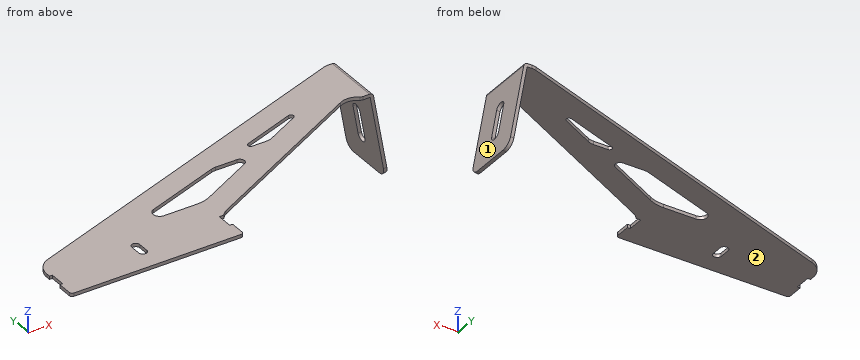
Autodesk Inventor part; units mm, degrees
ref_plane "工作平面1" through (65, 2, 0) normal (-1, 0, 0) x (0, 0, 1)
ref_plane "YZ Plane" through (0, 0, 0) normal (1, 0, 0) x (0, 1, 0)
ref_plane "XZ Plane" through (0, 0, 0) normal (0, 1, 0) x (-1, 0, 0)
sketch "草圖1" plane through (0, 0, 0) normal (0, 0, 1) x (1, 0, 0)
  line L0 (0, 0) -> (-7.8042, 0) construction
  line L1 (0, 0) -> (0, -16.694) construction
  line L2 (0, 2) -> (0, 13)
  line L3 (286, 136.6319) -> (286, 93.6319)
  line L4 (130, 19.7875) -> (130, 13) construction
  line L5 (128, 0) -> (2, 0)
  line L6 (286, 136.6319) -> (344, 136.6319)
  line L7 (351, 129.6319) -> (351, 100.6319)
  line L8 (344, 93.6319) -> (286, 93.6319)
  line L9 (308, 119.1319) -> (330, 119.1319)
  arc A0 (330, 111.1319) -> (330, 119.1319) centre (330, 115.1319) ccw
  line L10 (330, 111.1319) -> (308, 111.1319)
  arc A1 (308, 119.1319) -> (308, 111.1319) centre (308, 115.1319) ccw
  arc A2 (10.0615, 42.1637) -> (0, 28) centre (15, 28) ccw
  line L11 (10.0615, 42.1637) -> (279.401, 136.0744)
  line L12 (282.6934, 136.6319) -> (286, 136.6319)
  line L13 (286, 93.6319) -> (281, 93.6319)
  line L14 (265.3146, 95.4972) -> (135.4256, 28.6799)
  arc A3 (351, 129.6319) -> (344, 136.6319) centre (344, 129.6319) ccw
  arc A4 (344, 93.6319) -> (351, 100.6319) centre (344, 100.6319) ccw
  arc A5 (279.174, 94.2516) -> (281, 93.6319) centre (281, 96.6319) ccw
  arc A6 (279.174, 94.2516) -> (265.3146, 95.4972) centre (271.2613, 83.9371) ccw
  arc A7 (282.6934, 136.6319) -> (279.401, 136.0744) centre (282.6934, 126.6319) ccw
  arc A8 (135.4256, 28.6799) -> (131.466, 25) centre (140, 19.7875) ccw
  line L15 (0, 25) -> (2.15, 25)
  line L16 (2.15, 25) -> (2.15, 13)
  line L17 (2.15, 13) -> (0, 13)
  line L18 (0, 13) -> (0, 25) construction
  line L19 (65, 0) -> (65, 25) construction
  line L20 (131.466, 25) -> (127.85, 25)
  line L21 (127.85, 25) -> (127.85, 13)
  line L22 (127.85, 13) -> (130, 13)
  line L23 (130, 13) -> (130, 19.7875) construction
  arc A9 (0, 2) -> (2, 0) centre (2, 2) ccw
  arc A10 (128, 0) -> (130, 2) centre (128, 2) ccw
  line L24 (0, 13) -> (0, 25) construction
  line L25 (0, 25) -> (0, 28)
  line L26 (130, 19.7875) -> (130, 25) construction
  line L27 (130, 13) -> (130, 2)
  line L28 (123.9345, 45) -> (99.3585, 45)
  line L29 (157.566, 75) -> (173.8509, 75)
  line L30 (97.7123, 54.7212) -> (154.2737, 74.4425)
  line L31 (175.452, 68.3877) -> (135.3705, 47.769)
  arc A11 (175.452, 68.3877) -> (173.8509, 75) centre (173.8509, 71.5) ccw
  arc A12 (97.7123, 54.7212) -> (99.3585, 45) centre (99.3585, 50) ccw
  arc A13 (123.9345, 45) -> (135.3705, 47.769) centre (123.9345, 70) ccw
  arc A14 (157.566, 75) -> (154.2737, 74.4425) centre (157.566, 65) ccw
  line L32 (189.9693, 86.8885) -> (229.5263, 100.6808)
  line L33 (231.0996, 97.0139) -> (206.0106, 84.1076)
  line L34 (201.4362, 83) -> (190.6278, 83)
  arc A15 (231.0996, 97.0139) -> (229.5263, 100.6808) centre (230.1847, 98.7923) ccw
  arc A16 (201.4362, 83) -> (206.0106, 84.1076) centre (201.4362, 93) ccw
  arc A17 (189.9693, 86.8885) -> (190.6278, 83) centre (190.6278, 85) ccw
  arc A18 (131.466, 25) -> (130, 19.7875) centre (140, 19.7875) ccw construction
  line L35 (68, 25) -> (68, 17)
  arc A19 (62, 17) -> (68, 17) centre (65, 17) ccw
  line L36 (62, 17) -> (62, 25)
  arc A20 (68, 25) -> (62, 25) centre (65, 25) ccw
  point P0 (130, 0)
  point P1 (351, 136.6319)
  point P2 (351, 93.6319)
  point P3 (130, 25.8889)
  point P4 (281, 136.6319)
  point P5 (281, 93.6319)
  point P6 (281, 103.5661)
  point P7 (0, 10.2)
  point P8 (130, 28)
  point P9 (130, 10.2)
  dimension "d0" = 130
  dimension "d1" = 136.6319
  dimension "d2" = 43
  dimension "d3" = 65
  dimension "d4" = 8
  dimension "d5" = 30
  dimension "d7" = 18
  dimension "d8" = 286
  dimension "d17" = 21.5
  dimension "d20" = 15
  dimension "d21" = 28
  dimension "d23" = 5
  dimension "d24" = 7
  dimension "d26" = 3
  dimension "d29" = 13
  dimension "d30" = 5
  dimension "d31" = 10
  dimension "d32" = 10
  dimension "d33" = 8
  dimension "d39" = 12
  dimension "d41" = 13
  dimension "d42" = 2
  dimension "d45" = 45
  dimension "d46" = 17
  dimension "d47" = 17
  dimension "d48" = 30
  dimension "d49" = 3.5
  dimension "d50" = 5
  dimension "d51" = 25
  dimension "d52" = 10
  dimension "d53" = 8
  dimension "d54" = 2
  dimension "d55" = 10
  dimension "d56" = 2
  dimension "d57" = 19.7875
  dimension "d60" = 6
  dimension "d61" = 8
  dimension "d63" = 17
  dimension "d64" = 19.222
  dimension "d65" = 125.7
extrude "擠出1" add sketch "草圖1" along normal blind 2.5
bend part "折彎零件1" radius 0.5 angle 80 line through (286, 136.6319, 0) along (0, -1, 0) centre toward (0, 0, -1) moving side (1, 0, 0) both sides no
ref_plane "工作平面1" through (65, 2, 0) normal (-1, 0, 0) x (0, 0, 1)
properties part number "0 零件" material "不鏽鋼SUS-HL(砂紋)"
For this review, take the finished solid that the model builds, in its own axes (mm). Face numbers are marked on the shaded views. A direction names the side the tool comes from. Coordinates: 2 decimals unless noted, no trailing zeros. Order: outer loops, then holes, each group sorted by start corner. A loop starts at its lowest first (then second) coordinate and runs counter-clockwise, first axis right, second up. Notation, with made-up numbers: (-7, 49.25) -> (32, 49.25) arc R11 cw to (32, 64.25) -> close; hole circle Ø11 at (56, 59). An arc over 180 degrees is marked (long way). Return JSON: item names as keys, results as strings.
1. We need section A-A on z = -36. Write out the cut boundary in (x, y), and give its area (4 significant figures).
Answer block:
{"outline": "(292.77, 93.63) -> (295.31, 93.63) -> (295.31, 111.13) -> (292.77, 111.13) -> close; (292.77, 119.13) -> (295.31, 119.13) -> (295.31, 136.63) -> (292.77, 136.63) -> close", "area": "88.85 mm²"}
2. We need section B-B on x = 65. Write out the cut boundary in (y, z), and give its area (3 significant figures).
Answer block:
{"outline": "(0, 0) -> (14, 0) -> (14, 2.5) -> (0, 2.5) -> close; (28, 0) -> (61.32, 0) -> (61.32, 2.5) -> (28, 2.5) -> close", "area": "118 mm²"}
3. Machinability: for the marked faces 1 and 2, which of the approach directions +Z, -Z, +X, -X, +Y, -Y give a long, thin tool a straight path to every point of the face, cutting with its end or side? Answer none if there is none.
Answer block:
{"face 1": "+Z, +X, +Y, -Y", "face 2": "-Z, -X, +Y, -Y"}
4. We need section D-D on y = 103.5. Write out the cut boundary in (x, z).
Answer block:
{"outline": "(185.98, 0) -> (286, 0) arc R0.5 cw to (286.49, -0.41) -> (297.66, -63.74) -> (300.12, -63.3) -> (288.95, 0.02) arc R3 ccw to (286, 2.5) -> (185.98, 2.5) -> close"}
5. We need section C-C on y = 125. Write out the cut boundary in (x, z), and give its area (3 significant figures).
Answer block:
{"outline": "(247.64, 0) -> (286, 0) arc R0.5 cw to (286.49, -0.41) -> (297.66, -63.74) -> (300.12, -63.3) -> (288.95, 0.02) arc R3 ccw to (286, 2.5) -> (247.64, 2.5) -> close", "area": "263 mm²"}
6. For pin 1 Ø1.9 at (x, z) = (292, -27.5) entering from -Y; pin 2 Ø3 at (x, z) = (116, 1) entering from +Y; pin 3 Ø1.2 at (x, z) = (129, 2) entering from -Y; pin 4 Ø7 at (x, z) = (294.5, -29) entering from +Y, all flat-tipped, find the tip position at first contact; note any pin that passes through.
Answer block:
{"pin 1": "y = 93.63", "pin 2": "y = 79.62", "pin 3": "y = 0.04", "pin 4": "y = 136.63"}
7. For line 1 (Z direction, x = 209.5, y = 73); line 2 (X direction, y = 97, z = -31); line 3 (X direction, y = 102, z = -46), list the stretches that pass through material, from the lowest coordinate up. Write a range as from..to.
Answer block:
{"line 1": "0..2.5", "line 2": "291.89..294.42", "line 3": "294.53..297.07"}
